from build123d import *

# Parameters (mm, degrees)
SZKIC1_W                    = 100
SZKIC1_H                    = 100
DODANIE_WYCI_GNI_CIE1_DEPTH = 4
DODANIE_WYCI_GNI_CIE4_DEPTH = 196


with BuildPart() as part:
    # Szkic1 → Dodanie-wyciągnięcie1 (new body)
    with BuildSketch(Plane.XY):
        with Locations((-50, 50)):
            Rectangle(SZKIC1_W, SZKIC1_H)
        with Locations((50, 50)):
            Rectangle(SZKIC1_W, SZKIC1_H)
        with Locations((50, -50)):
            Rectangle(SZKIC1_W, SZKIC1_H)
        with Locations((-50, -50)):
            Rectangle(SZKIC1_W, SZKIC1_H)
    extrude(amount=DODANIE_WYCI_GNI_CIE1_DEPTH)

    # Szkic2 → Dodanie-wyciągnięcie4 (add)
    with BuildSketch(Plane.XY.offset(4)):
        Polygon((3, 100), (0, 100), (-3, 100), (100, -3), (100, 0), (100, 3), align=None)
    extrude(amount=DODANIE_WYCI_GNI_CIE4_DEPTH)


solid = part.part
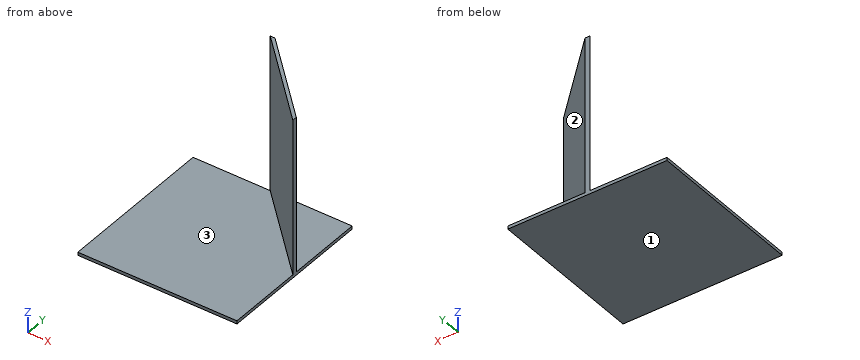
For this review, take the finished solid that the model builds, in its own axes (mm). Face numbers are marked on the shaded views. A direction names the side the tool comes from. Round coordinates to 2 decimals unless told otherwise and drop trailing zeros. Order: outer loops, then holes, each group sorted by start corner. A loop starts at its lowest first (then second) coordinate and runs counter-clockwise, first axis right, second up. Notation, with made-up numbers: (48.5, -6) -> (80.5, -6) arc R24 cw to (80.5, 30) -> close; hole circle Ø9 at (18.25, 24). An arc over 180 degrees is marked (long way). Put each result on its own line as item: value.
Q1. Insertion check: pin 1 Ø6 at (x, y) = (3.5, 51) entering from +Z; pin 2 Ø1.5 at (x, z) = (7, 82.5) entering from +Y; pin 3 Ø12 at (x, z) = (45, 28) entering from -Y. Each pin has a flat end and moves straight along its axis. Give the tip position at first contact, or say it passes through.
Check result:
pin 1: z = 4
pin 2: y = 96.75
pin 3: y = 46
Q2. Add section B-B on x = 59.5. Write out the cut boundary in (y, z).
Check result:
outline: (-100, 0) -> (100, 0) -> (100, 4) -> (43.5, 4) -> (43.5, 200) -> (37.5, 200) -> (37.5, 4) -> (-100, 4) -> close
Q3. Add section C-C on z = 152. Write out the cut boundary in (x, y), plus the area to 3 significant figures.
Check result:
outline: (-3, 100) -> (100, -3) -> (100, 3) -> (3, 100) -> close
area: 600 mm2
Q4. Machinability: for the marked faces 1, 2 and 3, which of the approach directions +Z, -Z, +X, -X, +Y, -Y give a long, thin tool a straight path to every point of the face, cutting with its end or side? Answer none if there is none.
Check result:
face 1: -Z, +X, -X, +Y, -Y
face 2: +Z, +X, +Y
face 3: +Z, -X, -Y
Q5. Add section D-D on y = -87. Write out the cut boundary in (x, z), plus the area to 3 significant figures.
Check result:
outline: (-100, 0) -> (100, 0) -> (100, 4) -> (-100, 4) -> close
area: 800 mm2
Q6. For probe 1 along Z at (x, y) = (-45, -73); probe 2 along Y at (x, z) = (50, 87); probe 3 along Y at (x, z) = (68, 108.5), list the stretches that pass through material, from the lowest coordinate up. Write a range as [from, to].
Check result:
probe 1: [0, 4]
probe 2: [47, 53]
probe 3: [29, 35]
Q7. Add section A-A on y = 72. Write out the cut boundary in (x, z).
Check result:
outline: (-100, 0) -> (100, 0) -> (100, 4) -> (31, 4) -> (31, 200) -> (25, 200) -> (25, 4) -> (-100, 4) -> close
